Read the model definition and answer for the solid it produces. Units are mm, in the model's axes. Face numbers are marked on the shaded views. A direction names the side the tool comes from. Give positions to 0.01 mm unless a question says otherwise; leave off trailing zeros. Order: outer loops, then holes, each group sorted by start corner. A loop starts at its lowest first (then second) coordinate and runs counter-clockwise, first axis right, second up.
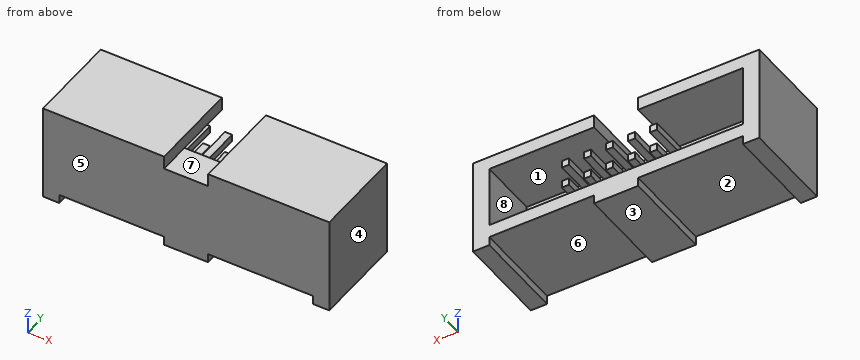
```python
from build123d import *

# Parameters (mm, degrees)
SKETCH1_W               = 16.51
SKETCH1_H               = 5.08
BOSS_EXTRUDE1_DEPTH     = 5.33
SKETCH2_W               = 14.63
SKETCH2_H               = 3.556
CUT_EXTRUDE1_DEPTH      = 3.45
SKETCH4_W               = 0.94
SKETCH4_H               = 5.33
SKETCH4_W_2             = 1.27
BOSS_EXTRUDE2_DEPTH     = 0.51
SKETCH5_W               = 1.27
SKETCH5_H               = 5.33
CUT_EXTRUDE2_DEPTH      = 0.762
SKETCH6_W               = 0.41
SKETCH6_H               = 0.41
BOSS_EXTRUDE3_DEPTH     = 3.05
LPATTERN1_COUNT         = 3
LPATTERN1_PITCH         = 1.27
LPATTERN1_COL_COUNT     = 3
LPATTERN1_COL_PITCH     = 1.27
MIRROR2_COPY_1_SKETCH_W = 0.41
MIRROR2_COPY_1_SKETCH_H = 0.41
MIRROR2_COPY_1_DEPTH    = 3.05
MIRROR2_COPY_2_SKETCH_W = 0.41
MIRROR2_COPY_2_SKETCH_H = 0.41
MIRROR2_COPY_2_DEPTH    = 3.05
MIRROR2_COPY_3_SKETCH_W = 0.41
MIRROR2_COPY_3_SKETCH_H = 0.41
MIRROR2_COPY_3_DEPTH    = 3.05
MIRROR2_COPY_4_SKETCH_W = 0.41
MIRROR2_COPY_4_SKETCH_H = 0.41
MIRROR2_COPY_4_DEPTH    = 3.05


with BuildPart() as part:
    # Sketch1 → Boss-Extrude1 (new body)
    with BuildSketch(Plane(origin=(0, 0, 0), x_dir=(1, 0, 0), z_dir=(0, 1, 0))):
        Rectangle(SKETCH1_W, SKETCH1_H)
    extrude(amount=BOSS_EXTRUDE1_DEPTH)

    # Sketch2 → Cut-Extrude1 (cut)
    with BuildSketch(Plane(origin=(0, 5.33, 0), x_dir=(1, 0, 0), z_dir=(0, 1, 0))):
        Rectangle(SKETCH2_W, SKETCH2_H)
    cut_extrude1 = extrude(amount=-CUT_EXTRUDE1_DEPTH, mode=Mode.SUBTRACT)

    # Sketch4 → Boss-Extrude2 (add)
    with BuildSketch(Plane(origin=(0, 0, -2.54), x_dir=(-1, 0, 0), z_dir=(0, 0, -1))):
        with Locations((-7.785, 2.665)):
            Rectangle(SKETCH4_W, SKETCH4_H)
        with Locations((-0.635, 2.665)):
            Rectangle(SKETCH4_W_2, SKETCH4_H)
    boss_extrude2 = extrude(amount=BOSS_EXTRUDE2_DEPTH)

    # Sketch5 → Cut-Extrude2 (cut)
    with BuildSketch(Plane.XY.offset(2.54)):
        with Locations((0.635, 2.665)):
            Rectangle(SKETCH5_W, SKETCH5_H)
    cut_extrude2 = extrude(amount=-CUT_EXTRUDE2_DEPTH, mode=Mode.SUBTRACT)

    # Mirror1: Cut-Extrude1, Boss-Extrude2, Cut-Extrude2 across plane
    add(cut_extrude1.mirror(Plane(origin=(0, 0, 0), x_dir=(0, 0, 1), z_dir=(1, 0, 0))), mode=Mode.SUBTRACT)
    add(boss_extrude2.mirror(Plane(origin=(0, 0, 0), x_dir=(0, 0, 1), z_dir=(1, 0, 0))))
    add(cut_extrude2.mirror(Plane(origin=(0, 0, 0), x_dir=(0, 0, 1), z_dir=(1, 0, 0))), mode=Mode.SUBTRACT)

    # Sketch6 → Boss-Extrude3 (add)
    with BuildSketch(Plane(origin=(0, 1.88, 0), x_dir=(1, 0, 0), z_dir=(0, 1, 0))):
        with Locations((0.635, -0.635)):
            Rectangle(SKETCH6_W, SKETCH6_H)
    boss_extrude3 = extrude(amount=BOSS_EXTRUDE3_DEPTH)

    # LPattern1: Boss-Extrude3 ×3
    with Locations(*[(i * LPATTERN1_PITCH, 0, 0) for i in range(1, LPATTERN1_COUNT)]):
        add(boss_extrude3)

    # LPattern1 col: Boss-Extrude3 ×3
    with Locations(*[(-i * LPATTERN1_COL_PITCH, 0, 0) for i in range(1, LPATTERN1_COL_COUNT)]):
        add(boss_extrude3)

    # Mirror2: Boss-Extrude3 across plane
    add(boss_extrude3.mirror(Plane.XY))

    # Mirror2 copy 1 sketch → Mirror2 copy 1 (add)
    with BuildSketch(Plane(origin=(1.27, 1.88, 0), x_dir=(1, 0, 0), z_dir=(0, 1, 0))):
        with Locations((0.635, 0.635)):
            Rectangle(MIRROR2_COPY_1_SKETCH_W, MIRROR2_COPY_1_SKETCH_H)
    extrude(amount=MIRROR2_COPY_1_DEPTH)

    # Mirror2 copy 2 sketch → Mirror2 copy 2 (add)
    with BuildSketch(Plane(origin=(2.54, 1.88, 0), x_dir=(1, 0, 0), z_dir=(0, 1, 0))):
        with Locations((0.635, 0.635)):
            Rectangle(MIRROR2_COPY_2_SKETCH_W, MIRROR2_COPY_2_SKETCH_H)
    extrude(amount=MIRROR2_COPY_2_DEPTH)

    # Mirror2 copy 3 sketch → Mirror2 copy 3 (add)
    with BuildSketch(Plane(origin=(-1.27, 1.88, 0), x_dir=(1, 0, 0), z_dir=(0, 1, 0))):
        with Locations((0.635, 0.635)):
            Rectangle(MIRROR2_COPY_3_SKETCH_W, MIRROR2_COPY_3_SKETCH_H)
    extrude(amount=MIRROR2_COPY_3_DEPTH)

    # Mirror2 copy 4 sketch → Mirror2 copy 4 (add)
    with BuildSketch(Plane(origin=(-2.54, 1.88, 0), x_dir=(1, 0, 0), z_dir=(0, 1, 0))):
        with Locations((0.635, 0.635)):
            Rectangle(MIRROR2_COPY_4_SKETCH_W, MIRROR2_COPY_4_SKETCH_H)
    extrude(amount=MIRROR2_COPY_4_DEPTH)


solid = part.part
```
1) A tool of negligible diameter and unlimited length cuts with its end or side. For the marked faces 5, 6, 7 and 8, from which of +Z, -Z, +X, -X, +Y, -Y can it reach the whole face along a straight path? Write none if from no direction.
Final values:
face 5: +Z, -Z, +X, -X, -Y
face 6: -Z, +Y, -Y
face 7: +Z, +Y, -Y
face 8: +Y
2) For a pull along X with two mould halves and no side action, classify the marked faces 1, 2, 3 and 4 as released by +X, released by -X, zero draft, split by the parting line, or undercut.
Final values:
face 1: undercut
face 2: undercut
face 3: zero draft
face 4: released by +X
3) The part is cut by section A-A on x = -0.25. Determine the outline of the cut face in (y, z), and give its area (3 significant figures).
Final values:
outline: (0, -3.05) - (5.33, -3.05) - (5.33, -1.78) - (1.88, -1.78) - (1.88, 1.78) - (0, 1.78) - close
area: 13.5 mm2
4) The part is cut by section D-D on y = 0.7. Determine the outline of the cut face in (x, z) (3 decimals), and give its area (3 significant figures).
Final values:
outline: (-8.255, -3.05) - (-7.315, -3.05) - (-7.315, -2.54) - (-1.27, -2.54) - (-1.27, -3.05) - (1.27, -3.05) - (1.27, -2.54) - (7.315, -2.54) - (7.315, -3.05) - (8.255, -3.05) - (8.255, 2.54) - (1.27, 2.54) - (1.27, 1.778) - (-1.27, 1.778) - (-1.27, 2.54) - (-8.255, 2.54) - close
area: 84.2 mm2
5) Consider L1, parallel to X at y = 0.85, z = -2.7 (3 decimals); L2, parallel to X at y = 3.7, z = -1.2 (3 decimals); L3, parallel to Z at x = -3.5, y = 3. Determine where each line is inside the solid, lowest interval first.
Final values:
L1: x = -8.255 to -7.315, -1.27 to 1.27, 7.315 to 8.255
L2: x = -8.255 to -7.315, 7.315 to 8.255
L3: z = -2.54 to -1.78, 1.78 to 2.54
6) Given pin 1 (0.9 mm diameter, centred on x = 0, y = 1, fed in from +Z); pin 2 (1.5 mm diameter, centred on x = 5.5, y = 3, fed in from -Z); pin 3 (1 mm diameter, centred on x = -4, z = -0.5, fed in from -Y), each flat-ended and moving along its own axis, determine where each tip first touches the part or whether it passes through.
Final values:
pin 1: stops at z = 1.78
pin 2: stops at z = -2.54
pin 3: stops at y = 0
7) The part is cut by section B-B on y = 3.35. Count the separate pieces of the cut face and the enclosed holes in it, and give its area (3 significant figures).
Final values:
separate pieces: 11
enclosed holes: 0
area: 33.8 mm2
8) The part is cut by section C-C on z = -1.4. Determine the outline of the cut face in (x, y) (3 decimals).
Final values:
outline: (-8.255, 0) - (8.255, 0) - (8.255, 5.33) - (7.315, 5.33) - (7.315, 1.88) - (-7.315, 1.88) - (-7.315, 5.33) - (-8.255, 5.33) - close
